Geometry: see drawing. Coordinates: mm, zero at the bounding-box minimum. Give positions to 0.01 mm unless a question says otherwise; leave off trailing zeros. Loops run counter-clockwise (first coordinate to the right, second up) from the corner with the lowest first, then second, coordinate; pieces in that order, holes last. Notation, with made-up numbers: M 22.25,87.25 L 45.25,87.25 A22 ccw 45.25,116.25 Z; hole C -16,83.5 d3. An arc over 180 degrees is marked long. Put each result on its own line as item: value.
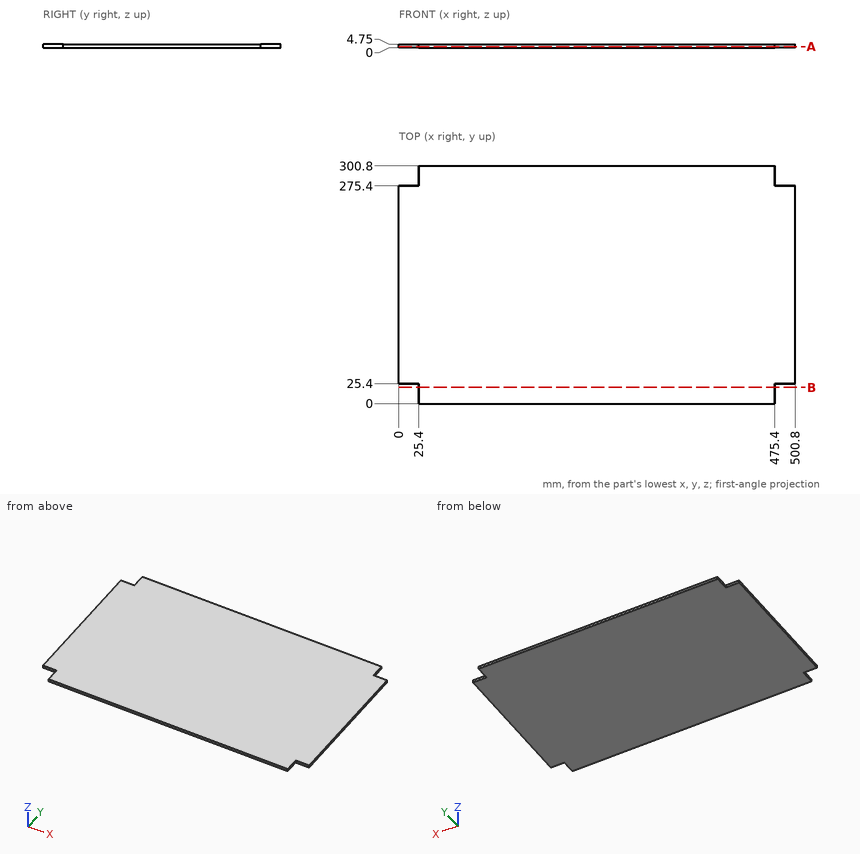
Item 1: Pin query (flat end, axial travel): pin 1 Ø2.5 at (x, z) = (488, 3) entering from +Y; pin 2 Ø2.5 at (y, z) = (18.5, 1.5) entering from +X; pin 3 Ø1.4 at (x, z) = (19, 3) entering from -Y. Return the tip coordinate at first contact, or that it passes through.
Output values:
pin 1: y = 275.4
pin 2: x = 475.4
pin 3: y = 25.4
Item 2: Section B-B on y = 20.5. Output: boundary loops of the cut face in (x, z).
Output values:
outline: M 25.4,0 L 475.4,0 L 475.4,4.75 L 25.4,4.75 Z
Item 3: Section A-A on z = 1.45. Output: boundary loops of the cut face in (x, y), then the cut area to 3 significant figures.
Output values:
outline: M 0,25.4 L 25.4,25.4 L 25.4,0 L 475.4,0 L 475.4,25.4 L 500.8,25.4 L 500.8,275.4 L 475.4,275.4 L 475.4,300.8 L 25.4,300.8 L 25.4,275.4 L 0,275.4 Z
area: 148,000 mm²
Item 4: Line query: probe 1 along Y at (x, z) = (22, 2.5). Output: solid intervals per line, ascending. Write a range as [from, to].
Output values:
probe 1: [25.4, 275.4]
